from build123d import *

# Parameters (mm, degrees)
SKETCH_R        = 2
SKETCH_R_2      = 3.25
SKETCH_R_3      = 3
SKETCH_R_4      = 1.625
SKETCH_W        = 10
SKETCH_H        = 5
PAD_DEPTH       = 8.25
POCKET_DEPTH    = 5.75
POCKET001_DEPTH = 8.5
POCKET002_DEPTH = 3.5
SKETCH006_W     = 5
SKETCH006_H     = 29
SKETCH006_W_2   = 16.5
SKETCH006_H_2   = 6
POCKET003_DEPTH = 7
CHAMFER_SIZE    = 4.9
CHAMFER001_SIZE = 4
FILLET_R        = 10
POCKET004_DEPTH = 3.5
SKETCH008_W     = 13
SKETCH008_H     = 9
POCKET005_DEPTH = 1
CHAMFER002_SIZE = 0.2


with BuildPart() as part:
    # Sketch → Pad (new body)
    with BuildSketch(Plane.XY):
        with BuildLine():
            Line((0, 20), (50, 20))
            Line((50, 20), (50, 0))
            Line((50, 0), (90, 0))
            ThreePointArc((90, 0), (75.3553389698, 35.3553391489), (39.9999997467, 50))
            Line((0, 50), (39.9999997467, 50))
            Line((-10, 60), (0, 50))
            Line((-15, 60), (-10, 60))
            Line((-15, 50), (-15, 60))
            Line((-40, 50), (-15, 50))
            Line((-50, 60), (-40, 50))
            Line((-106.4644660941, 60), (-50, 60))
            Line((-110, 56.4644660941), (-106.4644660941, 60))
            Line((-110, 28.5355339059), (-110, 56.4644660941))
            Line((-106.4644660941, 25), (-110, 28.5355339059))
            Line((-90, 25), (-106.4644660941, 25))
            Line((-69.14, 4.14), (-90, 25))
            Line((-55.5355339059, 4.14), (-69.14, 4.14))
            Line((-52, 0.6044660941), (-55.5355339059, 4.14))
            Line((-52, -6.4644660941), (-52, 0.6044660941))
            Line((-48.4644660941, -10), (-52, -6.4644660941))
            Line((-11.5355339059, -10), (-48.4644660941, -10))
            Line((-8, -6.4644660941), (-11.5355339059, -10))
            Line((-8, 0), (-8, -6.4644660941))
            Line((0, 0), (-8, 0))
            Line((0, 0), (0, 20))
        make_face()
        with Locations((56, 6)):
            Circle(SKETCH_R, mode=Mode.SUBTRACT)
        with Locations((-4, 16)):
            Circle(SKETCH_R, mode=Mode.SUBTRACT)
        with Locations((-8, 52)):
            Circle(SKETCH_R, mode=Mode.SUBTRACT)
        with Locations((-67, 10)):
            Circle(SKETCH_R, mode=Mode.SUBTRACT)
        with Locations((-78, 40)):
            Circle(SKETCH_R, mode=Mode.SUBTRACT)
        with Locations((-30, 27)):
            Circle(SKETCH_R_2, mode=Mode.SUBTRACT)
        with Locations((-46, 5)):
            Circle(SKETCH_R, mode=Mode.SUBTRACT)
        with Locations((-46, -5)):
            Circle(SKETCH_R, mode=Mode.SUBTRACT)
        with Locations((-14, 5)):
            Circle(SKETCH_R, mode=Mode.SUBTRACT)
        with Locations((-14, -5)):
            Circle(SKETCH_R, mode=Mode.SUBTRACT)
        with Locations((-52.5, 55.5)):
            Circle(SKETCH_R_3, mode=Mode.SUBTRACT)
        with Locations((-101.5, 47)):
            Circle(SKETCH_R_4, mode=Mode.SUBTRACT)
        with Locations((-78.5, 47)):
            Circle(SKETCH_R_4, mode=Mode.SUBTRACT)
        with Locations((-90, 34.5)):
            Rectangle(SKETCH_W, SKETCH_H, mode=Mode.SUBTRACT)
    extrude(amount=PAD_DEPTH)

    # SubtractivePipe: sweep along a path in Sketch001
    with BuildLine(Plane.XY.offset(8.25)) as subtractivepipe_path:
        Line((-70.9793119541, 1.9514059028), (-58.9653585777, 13.9653592792))
        ThreePointArc((-58.9653585777, 13.9653592792), (-52.5579976182, 18.2466208379), (-45.0000001258, 19.75))
        Line((-45.0000001258, 19.75), (39.9999998705, 19.75))
        ThreePointArc((39.9999998705, 19.75), (53.9653588826, 13.9653589742), (59.75, 0))
    # Sketch002 (on Face17 of Pad) → SubtractivePipe (sweep, cut)
    with BuildSketch(Plane(origin=(-32.5, -32.5, 0), x_dir=(0.7071067812, -0.7071067812, 0), z_dir=(-0.7071067812, -0.7071067812, 0))):
        Polygon((-80, 8.25), (-80, 1.75), (-78.75, 1.75), (-78.75, 4.75), (-70, 4.75), (-70, 8.25), align=None)
    sweep(path=subtractivepipe_path.line, mode=Mode.SUBTRACT)

    # Sketch003 (on DatumPlane) → Pocket (cut)
    with BuildSketch(Plane.XY.offset(8.25)):
        with BuildLine():
            ThreePointArc((-37.5, 48.2132034356), (-30, 4.5), (-22.5, 48.2132034356))
            Line((-22.5, 50.2132034356), (-22.5, 48.2132034356))
            Line((-37.5, 50.2132034356), (-22.5, 50.2132034356))
            Line((-37.5, 48.2132034356), (-37.5, 50.2132034356))
        make_face()
        Polygon((0, 50), (2, 48), (10, 48), (10, 50), align=None)
        Polygon((-40, 50), (-55, 50), (-65, 60), (-50, 60), align=None)
    extrude(amount=-POCKET_DEPTH, mode=Mode.SUBTRACT)

    # Sketch004 (on DatumPlane) → Pocket001 (cut)
    with BuildSketch(Plane.XY.offset(8.25)):
        with BuildLine():
            ThreePointArc((-49.0328663107, 15), (-30, 4.5), (-10.9671336893, 15))
            Line((-49.0328663107, 15), (-10.9671336893, 15))
        make_face()
    extrude(amount=-POCKET001_DEPTH, mode=Mode.SUBTRACT)

    # Sketch005 (on DatumPlane) → Pocket002 (cut)
    with BuildSketch(Plane.XY.offset(8.25)):
        Polygon((-41.375, 10), (-18.625, 10), (-18.625, 1), (-18.75, 1), (-18.75, -10), (-41.25, -10), (-41.25, 1), (-41.375, 1), align=None)
    extrude(amount=-POCKET002_DEPTH, mode=Mode.SUBTRACT)

    # Sketch006 → Pocket003 (cut)
    with BuildSketch(Plane.XY):
        with Locations((-107.5, 42.5)):
            Rectangle(SKETCH006_W, SKETCH006_H)
        with Locations((-96.25, 57)):
            Rectangle(SKETCH006_W_2, SKETCH006_H_2)
    extrude(amount=POCKET003_DEPTH, mode=Mode.SUBTRACT)

    # Chamfer
    chamfer_edges = [part.edges().sort_by_distance(p)[0] for p in [
        (-96.25, 54, 7),
        (-105, 42.5, 7),
    ]]
    chamfer(chamfer_edges, length=CHAMFER_SIZE)

    # Chamfer001
    chamfer001_edges = [part.edges().sort_by_distance(p)[0] for p in [
        (-90, 32, 0),
    ]]
    chamfer(chamfer001_edges, length=CHAMFER001_SIZE)

    # Fillet
    fillet_edges = [part.edges().sort_by_distance(p)[0] for p in [
        (-90, 32, 4),
    ]]
    fillet(fillet_edges, radius=FILLET_R)

    # Sketch007 (on DatumPlane) → Pocket004 (cut)
    with BuildSketch(Plane.XY.offset(8.25)):
        with BuildLine():
            ThreePointArc((87.7395276474, -1), (74.1160699454, 33.4089250273), (39.9999991, 47.75))
            Line((9.5, 47.75), (39.9999991, 47.75))
            Line((9.5, 50.25), (9.5, 47.75))
            Line((40, 50.25), (9.5, 50.25))
            ThreePointArc((90.2400487659, -1), (75.8839274606, 35.176785669), (40, 50.25))
            Line((87.7395276474, -1), (90.2400487659, -1))
        make_face()
    extrude(amount=-POCKET004_DEPTH, mode=Mode.SUBTRACT)

    # Sketch008 (on DatumPlane) → Pocket005 (cut)
    with BuildSketch(Plane.XY.offset(8.25)):
        with Locations((-90, 55.5)):
            Rectangle(SKETCH008_W, SKETCH008_H)
    extrude(amount=-POCKET005_DEPTH, mode=Mode.SUBTRACT)

    # Chamfer002
    chamfer002_edges = [part.edges().sort_by_distance(p)[0] for p in [
        (-85, 30, 0),
        (-85, 34.5, 0),
        (-90, 28, 0),
        (-90, 37, 0),
        (-95, 30, 0),
        (-95, 34.5, 0),
        (-4, 0, 0),
        (-8, -3.232233, 0),
        (-9.767767, -8.232233, 0),
        (-30, -10, 0),
        (-50.232233, -8.232233, 0),
        (-52, -2.93, 0),
        (-53.767767, 2.372233, 0),
        (-62.337767, 4.14, 0),
        (-79.57, 14.57, 0),
        (-98.232233, 25, 0),
        (-107.964466, 26.5, 0),
        (-107.232233, 28, 0),
        (-105, 42.5, 0),
        (-107.232233, 57, 0),
        (-107.964466, 58.5, 0),
        (-105.482233, 60, 0),
        (-104.5, 57, 0),
        (-96.25, 54, 0),
        (-88, 57, 0),
        (-69, 60, 0),
        (-45, 55, 0),
        (-27.5, 50, 0),
        (-15, 55, 0),
        (-12.5, 60, 0),
        (-5, 55, 0),
        (20, 50, 0),
        (75.355339, 35.355339, 0),
        (70, 0, 0),
        (50, 10, 0),
        (25, 20, 0),
        (0, 10, 0),
        (-80.125, 47, 0),
        (-55.5, 55.5, 0),
        (-80, 40, 0),
        (-48, -5, 0),
        (-16, -5, 0),
        (-30, 4.5, 0),
        (-30, 15, 0),
        (-16, 5, 0),
        (-48, 5, 0),
        (-69, 10, 0),
        (-33.25, 27, 0),
        (-10, 52, 0),
        (-6, 16, 0),
        (54, 6, 0),
        (-103.125, 47, 0),
    ]]
    chamfer(chamfer002_edges, length=CHAMFER002_SIZE)


solid = part.part
Design review of the part built by this model. Coordinates are the model's own, in mm. A direction names the side the tool comes from. Coordinates: 2 decimals unless noted, no trailing zeros. Loops run counter-clockwise (first coordinate to the right, second up) from the corner with the lowest first, then second, coordinate; pieces in that order, holes last. Notation, with made-up numbers: (41.5, -6.75) -> (53.5, -6.75) arc R29 cw to (53.5, 27.25) -> close; hole circle Ø6 at (-7, 0.25). An arc over 180 degrees is marked (long way). Use a Markdown table: item, result. Add a question column.
Item 1: We need section A-A, the plane x = 37. Write out the cut boundary in (y, z), and give its area (3 significant figures).
Item 2: We need section B-B, the plane y = 10. Count the separate pieces of the cut face and the enclosed holes in it, and give its area (3 significant figures).
Item 3: The part is to be moulded in two halves that separate along X. For faces 4 (the flat face through (-52, -3, 4)), 5 (the flat face through (-83.115, 28.255, 3.229)), 6 (the flat face through (-108, 57, 3)), say which applies: +X half, -X half, draft (parallel to the pull), parting line (faces both ways), or undercut.
Item 4: Clearance check with flat-ended pins moving along their axes: P1, Ø4, axis at x = 38.5, z = 1, coming from the -Y side; P2, Ø3.5, axis at x = -107, z = 3, coming from the -Y side; P3, Ø1.1, axis at y = 55.5, z = 7.5, coming from the +X side; P4, Ø2.5, axis at x = -78.5, y = 47, coming from the -Z side. State where each tip first meets the part, or that it passes through.
Item 5: Machinability: for faces 1 (the flat face through (-45, 55, 1)), 2 (the flat face through (-49.5, 54, 2.5)), 3 (the cylindrical face through (-63.68, 44.41, 4.95)), which of the approach directions +Z, -Z, +X, -X, +Y, -Y give a long, thin tool a straight path to every point of the face, cutting with its end or side? Answer none if there is none.
Item 6: Wall thickness on L1, parallel to Y at x = -30, z = 2; L2, parallel to Y at x = -30, z = 1.35; L3, parallel to X at y = 55.5, z = 1.5: over which ranges is each line inside the solid? List them lowest first. Write a range as from..to.
Numbers:
| question | item | result |
|---|---|---|
| 1 | outline | (20, 0.2) -> (20.2, 0) -> (49.8, 0) -> (50, 0.2) -> (50, 4.75) -> (48.18, 4.75) -> (48.18, 1.75) -> (46.93, 1.75) -> (46.93, 4.75) -> (38.18, 4.75) -> (38.18, 8.25) -> (20, 8.25) -> close |
| 1 | area | 202 mm^2 |
| 2 | separate pieces | 4 |
| 2 | enclosed holes | 0 |
| 2 | area | 618 mm^2 |
| 3 | face 4 | -X half |
| 3 | face 5 | undercut |
| 3 | face 6 | draft |
| 4 | P1 | stops at y = 20 |
| 4 | P2 | stops at y = 25 |
| 4 | P3 | stops at x = -4.95 |
| 4 | P4 | passes through |
| 5 | face 1 | +Z, -Z, +Y |
| 5 | face 2 | +Z, +Y |
| 5 | face 3 | +Z |
| 6 | L1 | y = -10..4.5, 15..23.75, 30.25..46.93, 48.18..50 |
| 6 | L2 | y = -10..4.5, 15..23.75, 30.25..50 |
| 6 | L3 | x = -105..-104.5, -88..-55.5, -49.5..-45.5, -15..-5.5 |
